Check sheet for the modelled part. Datum: model origin and axes. Units: mm. Face numbers are marked on the shaded views. A direction names the side the tool comes from. Coordinates: 2 decimals unless noted, no trailing zeros. Write each loop counter-clockwise with the first axis right and the second up, starting at its lowest first coordinate (ties: lowest second). Pieces come first, ordered by that corner, then holes. Notation, with made-up numbers: (47.5, 51.25) -> (89.5, 51.25) arc R35 ccw to (89.5, 90.25) -> close; hole circle Ø1 at (17.25, -19.75). An arc over 180 degrees is marked (long way). Put each result on its own line as item: value.
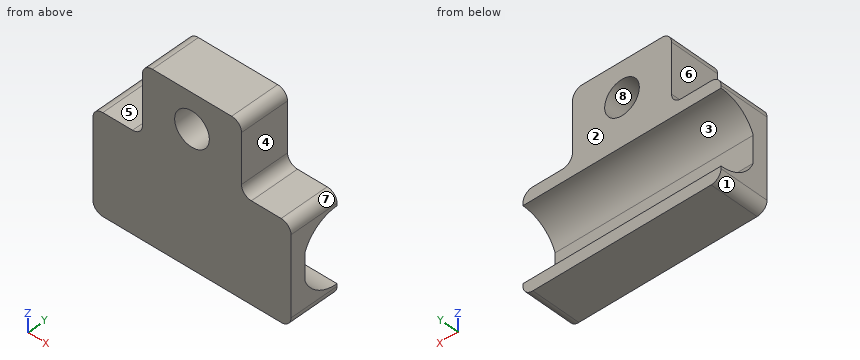
```python
from build123d import *

# Parameters (mm, degrees)
BOSS_EXTRUDE1_DEPTH = 10
SKETCH2_R           = 3.5
CUT_EXTRUDE1_DEPTH  = 10
CUT_EXTRUDE2_DEPTH  = 48.707441768
FILLET1_R           = 2


with BuildPart() as part:
    # Sketch1 → Boss-Extrude1 (new body)
    with BuildSketch(Plane(origin=(0, 0, 0), x_dir=(1, 0, 0), z_dir=(0, 1, 0))):
        Polygon((-10, -10), (-20, -10), (-20, 10), (20, 10), (20, -10), (10, -10), (10, -24), (-10, -24), align=None)
    extrude(amount=BOSS_EXTRUDE1_DEPTH)

    # Sketch2 → Cut-Extrude1 (cut)
    with BuildSketch(Plane(origin=(0, 10, 0), x_dir=(1, 0, 0), z_dir=(0, 1, 0))):
        with Locations(Location((0, -17, 0), (0, 0, 270))):
            Circle(SKETCH2_R)
    extrude(amount=-CUT_EXTRUDE1_DEPTH, mode=Mode.SUBTRACT)

    # Sketch3 → Cut-Extrude2 (cut, through all)
    with BuildSketch(Plane(origin=(20, 0, 0), x_dir=(0, 0, -1), z_dir=(1, 0, 0))):
        with BuildLine():
            Line((-2.692582404, 3), (2.692582404, 3))
            ThreePointArc((2.692582404, 3), (0, 17.5), (-2.692582404, 3))
        make_face()
    extrude(amount=-CUT_EXTRUDE2_DEPTH, mode=Mode.SUBTRACT)

    # Fillet1
    fillet1_edges = [part.edges().sort_by_distance(p)[0] for p in [
        (-20, 5, -10),
        (20, 5, -10),
        (20, 5, 10),
        (10, 5, 10),
        (10, 5, 24),
        (-10, 5, 24),
        (-10, 5, 10),
        (-20, 5, 10),
    ]]
    fillet(fillet1_edges, radius=FILLET1_R)


solid = part.part
```
Q1. Tool access check on the marked faces 1, 2, 3, 4 and 5. Record the directions out of +Z, -Z, +X, -X, +Y, -Y that give a thin tool (end or side, any length) a straight path to the whole face; none if there is none.
Recorded:
face 1: -Z, -X, +Y, -Y
face 2: +Z, -Z, +X, -X, +Y
face 3: +X, -X, +Y
face 4: +Z, +X, +Y, -Y
face 5: +Z, -X, +Y, -Y
Q2. Cross-section at D-D (y = 1). Record the cut outline in (x, z).
Recorded:
outline: (-20, -8) arc R2 ccw to (-18, -10) -> (18, -10) arc R2 ccw to (20, -8) -> (20, 8) arc R2 ccw to (18, 10) -> (12, 10) arc R2 cw to (10, 12) -> (10, 22) arc R2 ccw to (8, 24) -> (-8, 24) arc R2 ccw to (-10, 22) -> (-10, 12) arc R2 cw to (-12, 10) -> (-18, 10) arc R2 ccw to (-20, 8) -> close; hole circle Ø7 at (0, 17)
Q3. Mould release check, pull along Z, two halves, no side actions. Record for the marked faces 6, 7 and 8: released by +Z, released by -Z, zero draft, split by the parting line, or undercut.
Recorded:
face 6: zero draft
face 7: released by +Z
face 8: undercut
Q4. Cross-section at C-C (z = 17). Record the cut outline in (x, y), plus the area to 3 significant figures.
Recorded:
outline: (-10, 0) -> (-3.5, 0) -> (-3.5, 10) -> (-10, 10) -> close; (3.5, 0) -> (10, 0) -> (10, 10) -> (3.5, 10) -> close
area: 130 mm2
Q5. Depth check by flat-ended pin: P1, Ø2, axis at x = -8, z = 5.5, coming from the +Y side; P2, Ø6, axis at x = -3.5, z = 0.5, coming from the +Y side; P3, Ø3, axis at y = 7.5, z = 15, coming from the +X side. Enter the tip coordinate at first touch or a pass-through.
Recorded:
P1: stops at y = 6.26
P2: stops at y = 3.37
P3: stops at x = 10
Q6. Cross-section at A-A (x = 0). Record the cut outline in (y, z).
Recorded:
outline: (0, -10) -> (10, -10) -> (10, -7.5) arc R7.5 cw to (3, -2.69) -> (3, 2.69) arc R7.5 cw to (10, 7.5) -> (10, 13.5) -> (0, 13.5) -> close; (0, 20.5) -> (10, 20.5) -> (10, 24) -> (0, 24) -> close
Q7. Cross-section at B-B (y = 4.5). Record the cut outline in (x, z), plus the area to 3 significant figures.
Recorded:
outline: (-20, -8) arc R2 ccw to (-18, -10) -> (18, -10) arc R2 ccw to (20, -8) -> (20, -5.1) -> (-20, -5.1) -> close; (-20, 5.1) -> (20, 5.1) -> (20, 8) arc R2 ccw to (18, 10) -> (12, 10) arc R2 cw to (10, 12) -> (10, 22) arc R2 ccw to (8, 24) -> (-8, 24) arc R2 ccw to (-10, 22) -> (-10, 12) arc R2 cw to (-12, 10) -> (-18, 10) arc R2 ccw to (-20, 8) -> close; hole circle Ø7 at (0, 17)
area: 630 mm2
Q8. Material ranges on line 1 along X through (y, z) = (8, 17); line 2 along Z through (x, y) = (-3, 3.75); line 3 along Y through (x, z) = (-14.5, 1.5), recorded low to high.
Recorded:
line 1: x = -10 to -3.5, 3.5 to 10
line 2: z = -10 to -4.15, 4.15 to 15.2, 18.8 to 24
line 3: y = 0 to 3
